Geometry: final body of the model. Coordinates: model frame, mm. Face numbers are marked on the shaded views. A direction names the side the tool comes from. Round coordinates to 2 decimals unless told otherwise and drop trailing zeros. Loops run counter-clockwise (first coordinate to the right, second up) from the corner with the lowest first, then second, coordinate; pieces in that order, holes last. Notation, with made-up numbers: (43, 40) -> (59, 40) arc R20 ccw to (59, 53) -> close; hole circle Ø8 at (38, 46). An arc over 180 degrees is marked (long way). Answer in a Markdown table with one row per item.
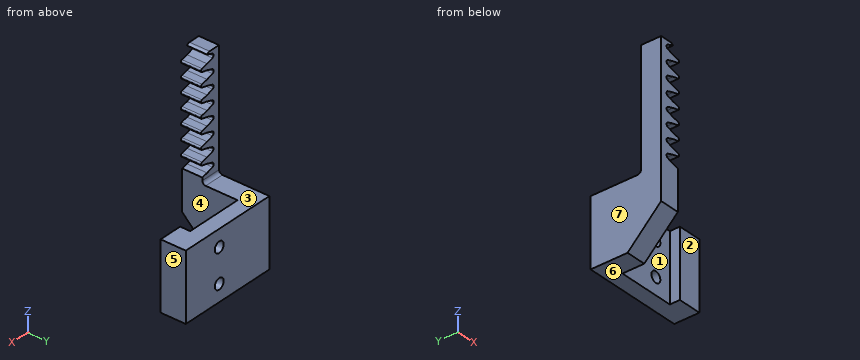
```python
from build123d import *

# Parameters (mm, degrees)
SKETCH1_W           = 30
SKETCH1_H           = 16
BOSS_EXTRUDE1_DEPTH = 20
CUT_EXTRUDE1_START  = -20
CUT_EXTRUDE1_DEPTH  = 20
SKETCH3_W           = 6
SKETCH3_H           = 10
BOSS_EXTRUDE2_DEPTH = 5
SKETCH9_R           = 1.6
CUT_EXTRUDE3_DEPTH  = 4.5
SKETCH11_W          = 8
SKETCH11_H          = 6
BOSS_EXTRUDE4_DEPTH = 40
FILLET1_R           = 1
CUT_EXTRUDE4_START  = -6
CUT_EXTRUDE4_DEPTH  = 6
SKETCH13_W          = 2
SKETCH13_H          = 6
BOSS_EXTRUDE5_DEPTH = 10
LPATTERN1_COUNT     = 8
LPATTERN1_PITCH     = 4.25
FILLET2_R           = 0.5
FILLET3_R           = 1
SKETCH14_W          = 2
SKETCH14_H          = 6
CUT_EXTRUDE5_DEPTH  = 17
CHAMFER9_SIZE       = 5


# Read off the part's stored shape, not the designer's step: Cut-Extrude1, Cut-Extrude4
with BuildPart() as part:
    # Sketch1 → Boss-Extrude1 (new body)
    with BuildSketch(Plane.XY):
        with Locations((15, -8)):
            Rectangle(SKETCH1_W, SKETCH1_H)
    extrude(amount=BOSS_EXTRUDE1_DEPTH)

    # Cut-Extrude1 outline → Cut-Extrude1 (cut)
    with BuildSketch(Plane.XY.offset(20).offset(CUT_EXTRUDE1_START)):
        Polygon((6, -4.5), (6, -16), (30, -16), (30, -7.5), (23, -7.5), (23, -4.5), align=None)
    extrude(amount=CUT_EXTRUDE1_DEPTH, mode=Mode.SUBTRACT)

    # Sketch3 → Boss-Extrude2 (add)
    with BuildSketch(Plane.XZ.offset(16)):
        with Locations((3, 10)):
            Rectangle(SKETCH3_W, SKETCH3_H)
    extrude(amount=BOSS_EXTRUDE2_DEPTH)

    # Sketch9 → Cut-Extrude3 (cut)
    with BuildSketch(Plane.XZ.offset(4.5)):
        with Locations(Location((18, 15, 0), (0, 0, 270))):
            Circle(SKETCH9_R)
        with Locations(Location((18, 5, 0), (0, 0, 270))):
            Circle(SKETCH9_R)
    extrude(amount=-CUT_EXTRUDE3_DEPTH, mode=Mode.SUBTRACT)

    # Sketch11 → Boss-Extrude4 (add)
    with BuildSketch(Plane.XY.offset(15)):
        with Locations((4, -18)):
            Rectangle(SKETCH11_W, SKETCH11_H)
    extrude(amount=BOSS_EXTRUDE4_DEPTH)

    # Fillet1
    fillet1_edges = [part.edges().sort_by_distance(p)[0] for p in [
        (3, -15, 20),
    ]]
    fillet(fillet1_edges, radius=FILLET1_R)

    # Cut-Extrude4 outline → Cut-Extrude4 (cut)
    with BuildSketch(Plane.XZ.offset(21).offset(CUT_EXTRUDE4_START)):
        Polygon((6.5, 51.5), (6.5, 50.75), (8, 50.75), (8, 55), (6.5, 55), (4.25, 54.5), (2, 53.75), (2, 52.75), (4.25, 52), align=None)
    cut_extrude4 = extrude(amount=CUT_EXTRUDE4_DEPTH, mode=Mode.SUBTRACT)

    # Sketch13 → Boss-Extrude5 (add)
    with BuildSketch(Plane(origin=(0, 0, 15), x_dir=(-1, 0, 0), z_dir=(0, 0, -1))):
        with Locations((-7, -18)):
            Rectangle(SKETCH13_W, SKETCH13_H)
    extrude(amount=BOSS_EXTRUDE5_DEPTH)

    # LPattern1: Cut-Extrude4 ×8
    with Locations(*[(0, 0, -i * LPATTERN1_PITCH) for i in range(1, LPATTERN1_COUNT)]):
        add(cut_extrude4, mode=Mode.SUBTRACT)

    # Fillet2
    # the kernel refuses this fillet: 0.5 mm, written as the material it adds along each edge
    with BuildSketch(Plane(origin=(2, -15, 52.75), x_dir=(0.9486832980505131, 0, -0.3162277660168398), z_dir=(0, -1, 0)), Plane(origin=(2, -15, 53.75), x_dir=(0, 0, -1), z_dir=(0, -1, 0)), Plane(origin=(2, -15, 48.5), x_dir=(0.9486832980505137, 0, -0.3162277660168381), z_dir=(0, -1, 0)), Plane(origin=(2, -15, 49.5), x_dir=(0, 0, -1), z_dir=(0, -1, 0)), Plane(origin=(2, -15, 44.25), x_dir=(0.9486832980505137, 0, -0.3162277660168381), z_dir=(0, -1, 0)), Plane(origin=(2, -15, 35.75), x_dir=(0.948683298050514, 0, -0.316227766016837), z_dir=(0, -1, 0)), Plane(origin=(2, -15, 36.75), x_dir=(0, 0, -1), z_dir=(0, -1, 0)), Plane(origin=(2, -15, 40), x_dir=(0.9486832980505137, 0, -0.31622776601683833), z_dir=(0, -1, 0)), Plane(origin=(2, -15, 41), x_dir=(0, 0, -1), z_dir=(0, -1, 0)), Plane(origin=(2, -15, 23), x_dir=(0.9486832980505137, 0, -0.31622776601683833), z_dir=(0, -1, 0)), Plane(origin=(2, -15, 24), x_dir=(0, 0, -1), z_dir=(0, -1, 0)), Plane(origin=(2, -15, 27.25), x_dir=(0.9486832980505135, 0, -0.3162277660168391), z_dir=(0, -1, 0)), Plane(origin=(2, -15, 28.25), x_dir=(0, 0, -1), z_dir=(0, -1, 0)), Plane(origin=(2, -15, 32.5), x_dir=(0, 0, -1), z_dir=(0, -1, 0)), Plane(origin=(2, -15, 31.5), x_dir=(0.9486832980505139, 0, -0.3162277660168378), z_dir=(0, -1, 0))) as fillet2_piece_1:
        with BuildLine():
            CenterArc((FILLET2_R * 0.720759220056, FILLET2_R), FILLET2_R, 198.434948823, 71.565051177)
            Line((-FILLET2_R * 0.227924077994, FILLET2_R * 0.683772233983), (0, 0))
            Line((0, 0), (FILLET2_R * 0.720759220056, 0))
        make_face()
    extrude(amount=6)
    with BuildSketch(Plane(origin=(2, -15, 45.25), x_dir=(0.948683298050513, 0, 0.31622776601684033), z_dir=(0, -1, 0))) as fillet2_piece_2:
        with BuildLine():
            CenterArc((FILLET2_R * 0.720759220056, -FILLET2_R), FILLET2_R, 90, 71.565051177)
            Line((-FILLET2_R * 0.227924077994, -FILLET2_R * 0.683772233983), (0, 0))
            Line((0, 0), (FILLET2_R * 0.720759220056, 0))
        make_face()
    extrude(amount=6)
    # the kernel refuses this fillet: 0.5 mm, written as the material it takes off along each edge
    with BuildSketch(Plane(origin=(6.5, -13.997285492, 33.75), x_dir=(-0.9761870601839541, 0, -0.21693045781865056), z_dir=(0, -1, 0)), Plane(origin=(6.5, -13.997285492, 34.5), x_dir=(0, 0, -1), z_dir=(0, -1, 0)), Plane(origin=(6.5, -13.997285492, 38), x_dir=(-0.9761870601839538, 0, -0.216930457818651), z_dir=(0, -1, 0)), Plane(origin=(6.5, -13.997285492, 38.75), x_dir=(0, 0, -1), z_dir=(0, -1, 0)), Plane(origin=(6.5, -13.997285492, 42.25), x_dir=(-0.9761870601839541, 0, -0.21693045781865006), z_dir=(0, -1, 0)), Plane(origin=(6.5, -13.997285492, 43), x_dir=(0, 0, -1), z_dir=(0, -1, 0)), Plane(origin=(6.5, -13.997285492, 46.5), x_dir=(-0.9761870601839537, 0, -0.21693045781865147), z_dir=(0, -1, 0)), Plane(origin=(6.5, -13.997285492, 47.25), x_dir=(0, 0, -1), z_dir=(0, -1, 0)), Plane(origin=(6.5, -13.997285492, 50.75), x_dir=(-0.9761870601839537, 0, -0.21693045781865147), z_dir=(0, -1, 0)), Plane(origin=(6.5, -13.997285492, 51.5), x_dir=(0, 0, -1), z_dir=(0, -1, 0)), Plane(origin=(6.5, -13.997285492, 25.25), x_dir=(-0.9761870601839521, 0, -0.21693045781865947), z_dir=(0, -1, 0)), Plane(origin=(6.5, -13.997285492, 26), x_dir=(0, 0, -1), z_dir=(0, -1, 0)), Plane(origin=(6.5, -13.997285492, 29.5), x_dir=(-0.9761870601839522, 0, -0.2169304578186585), z_dir=(0, -1, 0)), Plane(origin=(6.5, -13.997285492, 30.25), x_dir=(0, 0, -1), z_dir=(0, -1, 0))) as fillet2_2_piece_1:
        with BuildLine():
            CenterArc((FILLET2_R * 0.802171606366, -FILLET2_R), FILLET2_R, 90, 77.471192291)
            Line((-FILLET2_R * 0.174015453818, -FILLET2_R * 0.783069542181), (0, 0))
            Line((0, 0), (FILLET2_R * 0.802171606366, 0))
        make_face()
    extrude(amount=8.005429016, mode=Mode.SUBTRACT)

    # Fillet3
    # the kernel refuses this fillet: 1 mm, written as the material it takes off along each edge
    with BuildSketch(Plane(origin=(6.5, -7.209936491, 55), x_dir=(-0.9761870601839528, 0, -0.21693045781865575), z_dir=(0, -1, 0))) as fillet3_piece_1:
        with BuildLine():
            CenterArc((3.258754136, 0.300226243), FILLET3_R, 197.471192291, 60)
            Line((3.041823678, -0.675960817), (0, 0))
            Line((0, 0), (2.304886114, 0))
        make_face()
    extrude(amount=21.580127019, mode=Mode.SUBTRACT)

    # Sketch14 → Cut-Extrude5 (cut)
    with BuildSketch(Plane(origin=(0, 0, 5), x_dir=(-1, 0, 0), z_dir=(0, 0, -1))):
        with Locations((-7, -18)):
            Rectangle(SKETCH14_W, SKETCH14_H)
    extrude(amount=-CUT_EXTRUDE5_DEPTH, mode=Mode.SUBTRACT)

    # Chamfer9
    # the kernel refuses this chamfer: 5 mm, written as the material it adds along each edge
    # the kernel refuses this chamfer: 5 mm, written as the material it takes off along each edge
    with BuildSketch(Plane(origin=(18.85841494, -21, 5), x_dir=(0, -0.027495876610586393, 0.9996219169112968), z_dir=(-1, 0, 0))) as chamfer9_2_piece_1:
        Polygon((CHAMFER9_SIZE * 0.999621916911, CHAMFER9_SIZE * 0.0274958766106), (-CHAMFER9_SIZE * 0.0274958766106, CHAMFER9_SIZE * 0.999621916911), (0, 0), align=None)
    extrude(amount=31.71682988, mode=Mode.SUBTRACT)
    with BuildSketch(Plane(origin=(18.85841494, -16, 0), x_dir=(0, 0.9996219169112968, -0.027495876610586372), z_dir=(-1, 0, 0))) as chamfer9_2_piece_2:
        Polygon((CHAMFER9_SIZE * 0.999621916911, -CHAMFER9_SIZE * 0.0274958766106), (-CHAMFER9_SIZE * 0.0274958766106, -CHAMFER9_SIZE * 0.999621916911), (0, 0), align=None)
    extrude(amount=31.71682988, mode=Mode.SUBTRACT)


solid = part.part
```
Item 1: Cut plane A-A (z = 5). Output: boundary loops of the cut face in (x, y).
Answer:
| item | result |
|---|---|
| outline | (0, -16) -> (6, -16) -> (6, -4.5) -> (16.4, -4.5) -> (16.4, 0) -> (0, 0) -> close; (19.6, -4.5) -> (23, -4.5) -> (23, -7.5) -> (30, -7.5) -> (30, 0) -> (19.6, 0) -> close |
Item 2: Line query: probe 1 along X at (y, z) = (-2.35, 5); probe 2 along Z at (x, y) = (18.5, -1); probe 3 along Z at (x, y) = (23.25, -6.5). Output: solid intervals per line, ascending. Write a range as [from, to].
Answer:
| item | result |
|---|---|
| probe 1 | x = [0, 16.4], [19.6, 30] |
| probe 2 | z = [0, 3.48], [6.52, 13.48], [16.52, 20] |
| probe 3 | z = [0, 20] |
Item 3: Pin query (flat end, axial travel): pin 1 Ø7 at (x, z) = (4, 39) entering from +Y; pin 2 Ø8 at (x, y) = (3.5, -17) entering from +Z; pin 3 Ø6 at (x, y) = (7, -15.5) entering from +Z; pin 4 Ø5 at (x, z) = (15.5, 11.5) entering from -Y. Return the tip coordinate at first contact, or that it passes through.
Answer:
| item | result |
|---|---|
| pin 1 | stops at y = -15 |
| pin 2 | stops at z = 55 |
| pin 3 | stops at z = 54.79 |
| pin 4 | stops at y = -4.5 |
Item 4: Cut plane C-C (x = 18). Output: boundary loops of the cut face in (y, z).
Answer:
| item | result |
|---|---|
| outline | (-4.5, 0) -> (0, 0) -> (0, 3.4) -> (-4.5, 3.4) -> close; (-4.5, 6.6) -> (0, 6.6) -> (0, 13.4) -> (-4.5, 13.4) -> close; (-4.5, 16.6) -> (0, 16.6) -> (0, 20) -> (-4.5, 20) -> close |
Item 5: Cut plane B-B (y = -6.75). Output: boundary loops of the cut face in (x, z), then the cut area to 3 significant figures.
Answer:
| item | result |
|---|---|
| outline | (0, 0) -> (6, 0) -> (6, 20) -> (0, 20) -> close; (23, 0) -> (30, 0) -> (30, 20) -> (23, 20) -> close |
| area | 260 mm² |
Item 6: Reachability of the marked faces 1, 2 and 3 from +Z, -Z, +X, -X, +Y, -Y: full face, straight path, thin tool, end or side. Return the list, or none.
Answer:
| item | result |
|---|---|
| face 1 | +Z, -Z, -Y |
| face 2 | +Z, -Z, +X, -Y |
| face 3 | +Z, +X, -X, +Y |
Item 7: Cut plane D-D (y = -2). Output: boundary loops of the cut face in (x, z), then the cut area to 3 significant figures.
Answer:
| item | result |
|---|---|
| outline | (0, 0) -> (30, 0) -> (30, 20) -> (0, 20) -> close; hole circle Ø3.2 at (18, 5); hole circle Ø3.2 at (18, 15) |
| area | 584 mm² |
Item 8: Draft query along X for the marked faces 4, 5, 6 and 7. Return one class per face: pulls with the +X half, pulls with the -X half, needs draft (parallel to the pull), parting line crosses it, or undercut.
Answer:
| item | result |
|---|---|
| face 4 | undercut |
| face 5 | pulls with the +X half |
| face 6 | needs draft |
| face 7 | pulls with the -X half |
